```python
from build123d import *

# Parameters (mm, degrees)
F0_W     = 38.1
F0_H     = 38.1
F0_W_2   = 25.4
F0_H_2   = 25.4
F1_DEPTH = 203.2
F2_R     = 5.08
F5_DEPTH = 38.1


with BuildPart() as f1:
    # F0 (on Top) → F1 (new body)
    with BuildSketch(Plane.XY):
        Rectangle(F0_W, F0_H)
        Rectangle(F0_W_2, F0_H_2, mode=Mode.SUBTRACT)
    extrude(amount=F1_DEPTH)

    # F2
    f2_edges = [f1.edges().sort_by_distance(p)[0] for p in [
        (-19.05, 19.05, 101.6),
        (-19.05, -19.05, 101.6),
        (19.05, -19.05, 101.6),
        (19.05, 19.05, 101.6),
        (-12.7, 12.7, 101.6),
        (12.7, 12.7, 101.6),
        (12.7, -12.7, 101.6),
        (-12.7, -12.7, 101.6),
    ]]
    fillet(f2_edges, radius=F2_R)

    # F3: F1 across face


with BuildPart() as f1_1:
    add(f1.part)
    add(f1.part.mirror(Plane.XY.offset(203.2)))

    # F4 (on face) → F5 (cut, through all)
    with BuildSketch(Plane(origin=(-19.05, 0, 0), x_dir=(0, -1, 0), z_dir=(-1, 0, 0))):
        Polygon((19.05, 10.208864), (-19.05, 0), (19.05, 0), align=None)
    extrude(amount=-F5_DEPTH, mode=Mode.SUBTRACT)


solid = f1_1.part
```
Could you check a few things on this model? Use its own coordinates, in mm. A direction names the side the tool comes from. Round coordinates to 2 decimals unless told otherwise and drop trailing zeros. Loops run counter-clockwise (first coordinate to the right, second up) from the corner with the lowest first, then second, coordinate; pieces in that order, holes last. Notation, with made-up numbers: M -3,89 L 46,89 A7 cw 46,98 Z; hole C 73.25,35.25 d3. An arc over 180 degrees is marked long. Put each result on its own line as item: value.
Q1. For pin 1 (1.5 mm diameter, centred on x = -1.5, y = -14, fed in from -Z), with a flat end and sliding along its axis, tell me the tip position at first contact or that it passes through.
Check result:
pin 1: z = 8.65
Q2. Imagine slicing it at B-B (z = 49). Write out the boundary of the cut face in (x, y), then the cut area to 3 significant figures.
Check result:
outline: M -19.05,-13.97 A5.08 ccw -13.97,-19.05 L 13.97,-19.05 A5.08 ccw 19.05,-13.97 L 19.05,13.97 A5.08 ccw 13.97,19.05 L -13.97,19.05 A5.08 ccw -19.05,13.97 Z; hole M -12.7,-7.62 A5.08 ccw -7.62,-12.7 L 7.62,-12.7 A5.08 ccw 12.7,-7.62 L 12.7,7.62 A5.08 ccw 7.62,12.7 L -7.62,12.7 A5.08 ccw -12.7,7.62 Z
area: 806 mm2
Q3. Imagine slicing it at A-A (x = -4). Write out the boundary of the cut face in (y, z).
Check result:
outline: M -19.05,10.21 L -12.7,8.51 L -12.7,406.4 L -19.05,406.4 Z; M 12.7,1.7 L 19.05,0 L 19.05,406.4 L 12.7,406.4 Z
Q4. Thinking about a two-plate mould opening in X: for faces 3 (the face through (-19.05, 0, 207)), 4 (the face through (19.05, 0, 207)), 5 (the face through (12.7, 0, 208)), 6 (the face through (-13, 0, 406.4)), which applies, released by +X, released by -X, zero draft, split by the parting line, or undercut?
Check result:
face 3: released by -X
face 4: released by +X
face 5: undercut
face 6: zero draft
Q5. I need wall thicknesses on probe 1 along X at (y, z) = (-7.5, 373.5); probe 2 along Z at (x, y) = (-6, -14). Which ranges of each line are inside material? Lowest first, please.
Check result:
probe 1: -19.05 to -12.7, 12.7 to 19.05
probe 2: 8.86 to 406.4
Q6. On a 3-axis mill with a long thin cutter (end or side, diameter ignored), from which of +Z, -Z, +X, -X, +Y, -Y can I reach the whole of each face in a straight line? I mean faces 1 (the face through (0, 12.7, 207)), 2 (the face through (0, -19.05, 211)). Say none if no direction works.
Check result:
face 1: +Z, -Z
face 2: +Z, -Z, +X, -X, -Y
Q7. Imagine slicing it at C-C (y = 0.5). Write out the boundary of the cut face in (x, z).
Check result:
outline: M -19.05,4.97 L -12.7,4.97 L -12.7,406.4 L -19.05,406.4 Z; M 12.7,4.97 L 19.05,4.97 L 19.05,406.4 L 12.7,406.4 Z
